Check sheet for the modelled part. Datum: model origin and axes. Units: mm. Face numbers are marked on the shaded views. A direction names the side the tool comes from. Round coordinates to 2 decimals unless told otherwise and drop trailing zeros. Write each loop counter-clockwise with the first axis right and the second up, starting at its lowest first coordinate (ties: lowest second). Pieces come first, ordered by that corner, then holes. Notation, with made-up numbers: (34.25, -29) - (86.25, -29) arc R9 ccw to (86.25, -16) - close; hole circle Ø9 at (-21.75, 28.25). An arc over 180 degrees is marked (long way). Answer as a JSON object with one key per item and string values. Group by question number.
Item 1: Sectioned sample at C-C on x = 5.25. Record the boundary of the cut face in (y, z), plus the area to 3 significant figures.
Item 2: Set-up check for the marked faces 4, 5, 6, 7 and 8: record each of +Z, -Z, +X, -X, +Y, -Y from which the full face is reachable in a straight line by a thin tool's end or side.
Item 3: Sectioned sample at B-B on z = 13. Record the boundary of the cut face in (x, y), plus the area to 3 significant figures.
Item 4: Sectioned sample at D-D on x = -18. Record the boundary of the cut face in (y, z) (3 decimals), plus the area to 3 significant figures.
Item 5: Gauge pin test, flat ends, axial feed: P1, Ø2, axis at y = -5, z = 14.5, coming from the -X side; P2, Ø7, axis at x = -11, z = 13, coming from the -Y side; P3, Ø5.5, axis at x = -17, z = 7.5, coming from the -Y side; P4, Ø12.5, axis at x = 5.25, z = 13, coming from the +Y side. Record the tip position at first contact, or that the pin passes through.
Item 6: Release check for a two-part mould opening along Z. For the marked faces 1, 2 and 3 record: pulls with the +Z half, pulls with the -Z half, needs draft (parallel to the pull), parting line crosses it, or undercut.
Item 7: Sectioned sample at A-A on y = -9.5. Record the boundary of the cut face in (x, z), plus the area to 3 significant figures.
Item 8: Thickness scan on line 1 (X direction, y = -6.5, z = 13); line 2 (Z direction, x = 5.25, y = -6); line 3 (Z direction, x = 5.25, y = -2). Record the ranges inside material, lowest first.
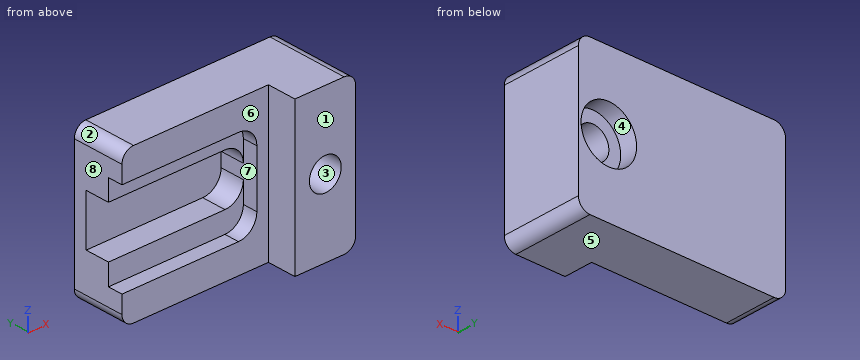
```python
from build123d import *

# Parameters (mm, degrees)
BOSS_EXTRUDE1_DEPTH             = 26
FILLET2_R                       = 2
CBORE_FOR_M5_SBHCS1_D           = 5.5
CBORE_FOR_M5_SBHCS1_CBORE_D     = 9.6
CBORE_FOR_M5_SBHCS1_CBORE_DEPTH = 3
SKETCH10_W                      = 8.75
SKETCH10_H                      = 4.2
SKETCH10_W_2                    = 16
SKETCH10_H_2                    = 2.55
CUT_EXTRUDE3_DEPTH              = 23.3
FILLET6_R                       = 3.175


with BuildPart() as part:
    # Sketch1 → Boss-Extrude1 (new body)
    with BuildSketch(Plane.XY):
        Polygon((-25.3, 0), (-25.3, -9), (0, -9), (0, -14), (10.5, -14), (10.5, 0), (0, 0), align=None)
    extrude(amount=BOSS_EXTRUDE1_DEPTH)

    # Fillet2
    fillet2_edges = [part.edges().sort_by_distance(p)[0] for p in [
        (10.5, -7, 26),
        (10.5, -7, 0),
        (-25.3, -4.5, 26),
        (-25.3, -4.5, 0),
    ]]
    fillet(fillet2_edges, radius=FILLET2_R)

    # CBORE for M5 SBHCS1 (through all)
    with Locations(Plane(origin=(0, 0, 0), x_dir=(1, 0, 0), z_dir=(0, 1, 0))):
        with Locations((5.25, -13)):
            CounterBoreHole(CBORE_FOR_M5_SBHCS1_D / 2, CBORE_FOR_M5_SBHCS1_CBORE_D / 2, CBORE_FOR_M5_SBHCS1_CBORE_DEPTH)

    # Sketch10 → Cut-Extrude3 (cut)
    with BuildSketch(Plane.ZY.offset(25.3)):
        with Locations((13, -4.35)):
            Rectangle(SKETCH10_W, SKETCH10_H)
        with Locations((13, -7.725)):
            Rectangle(SKETCH10_W_2, SKETCH10_H_2)
    extrude(amount=-CUT_EXTRUDE3_DEPTH, mode=Mode.SUBTRACT)

    # Fillet6
    fillet6_edges = [part.edges().sort_by_distance(p)[0] for p in [
        (-2, -7.725, 21),
        (-2, -7.725, 5),
        (-2, -4.35, 8.625),
        (-2, -4.35, 17.375),
    ]]
    fillet(fillet6_edges, radius=FILLET6_R)


solid = part.part
```
Completed:
{
 "1": {"outline": "(-14, 0) - (0, 0) - (0, 8.2) - (-3, 8.2) - (-3, 10.25) - (-14, 10.25) - close; (-14, 15.75) - (-3, 15.75) - (-3, 17.8) - (0, 17.8) - (0, 26) - (-14, 26) - close", "area": "275 mm²"},
 "2": {"face 4": "+Y", "face 5": "-Z, +X, -X, +Y, -Y", "face 6": "+Z, -Z, -X, -Y", "face 7": "-X, -Y", "face 8": "+Z, -Z, -X, +Y, -Y"},
 "3": {"outline": "(-25.3, -2.25) - (-2, -2.25) - (-2, -9) - (0, -9) - (0, -14) - (2.5, -14) - (2.5, -3) - (0.45, -3) - (0.45, 0) - (-25.3, 0) - close; (8, -14) - (10.5, -14) - (10.5, 0) - (10.05, 0) - (10.05, -3) - (8, -3) - close", "area": "128 mm²"},
 "4": {"outline": "(-9, 0) - (0, 0) - (0, 26) - (-9, 26) - (-9, 21) - (-6.45, 21) - (-6.45, 17.375) - (-2.25, 17.375) - (-2.25, 8.625) - (-6.45, 8.625) - (-6.45, 5) - (-9, 5) - close", "area": "156 mm²"},
 "5": {"P1": "x = -2.28", "P2": "y = -2.25", "P3": "y = -9", "P4": "y = 0"},
 "6": {"face 1": "needs draft", "face 2": "pulls with the +Z half", "face 3": "undercut"},
 "7": {"outline": "(0, 0) - (8.5, 0) arc R2 ccw to (10.5, 2) - (10.5, 24) arc R2 ccw to (8.5, 26) - (0, 26) - close; hole circle Ø5.5 at (5.25, 13)", "area": "248 mm²"},
 "8": {"line 1": "-2 to 2.5, 8 to 10.5", "line 2": "0 to 10.25, 15.75 to 26", "line 3": "0 to 8.2, 17.8 to 26"}
}
